Model file for the job. Use its own axes, mm. Round coordinates to 2 decimals unless told otherwise and drop trailing zeros. Loops run counter-clockwise (first coordinate to the right, second up) from the corner with the lowest first, then second, coordinate; pieces in that order, holes last. Notation, with made-up numbers: (59, 82) -> (91, 82) arc R13 ccw to (91, 103) -> close; hole circle Ø7 at (18.5, 48). An arc over 180 degrees is marked (long way). Use a Markdown table: item, result.
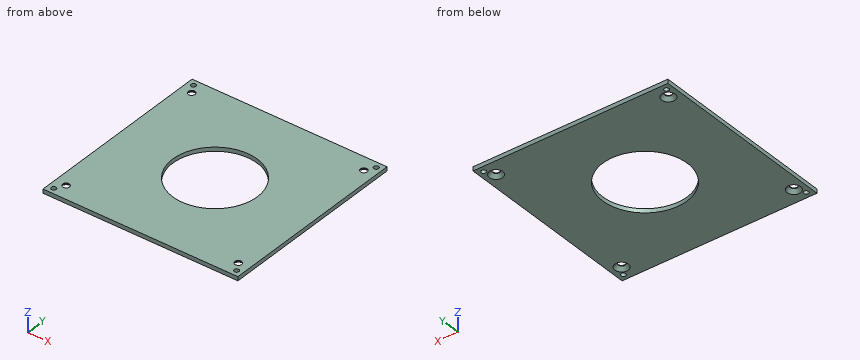
from build123d import *

# Parameters (mm, degrees)
PLATE_SKETCH_W                 = 97
PLATE_SKETCH_H                 = 95
PLATE_DEPTH                    = 2
M2_FOOT_SCREW_HOLES_DEPTH      = 136.786597277
M2_FOOT_SCREW_HOLES_DEPTH_BACK = 136.786597277
M2_FOOT_SCREW_HOLES_SKETCH_R   = 1.2
M3_STACK_ROD_HOLES_DEPTH       = 136.786597277
M3_STACK_ROD_HOLES_DEPTH_BACK  = 136.786597277
M3_STACK_ROD_HOLES_SKETCH_R    = 1.7
M3_COUNTERSINKS_SIZE           = 1.66
CAMERA_APERTURE_DEPTH          = 136.786597277
CAMERA_APERTURE_DEPTH_BACK     = 136.786597277
CAMERA_APERTURE_SKETCH_R       = 21


with BuildPart() as part:
    # Plate sketch → Plate (new body)
    with BuildSketch(Plane.XY):
        with Locations((48.5, 47.5)):
            Rectangle(PLATE_SKETCH_W, PLATE_SKETCH_H)
    extrude(amount=PLATE_DEPTH)

    # M2 foot screw holes sketch → M2 foot screw holes (cut, two sides: drawn at the far end of the back side and taken through both)
    with BuildSketch(Plane.XY.offset(-M2_FOOT_SCREW_HOLES_DEPTH_BACK)):
        with Locations((3, 3)):
            Circle(M2_FOOT_SCREW_HOLES_SKETCH_R)
        with Locations((94, 3)):
            Circle(M2_FOOT_SCREW_HOLES_SKETCH_R)
        with Locations((3, 92)):
            Circle(M2_FOOT_SCREW_HOLES_SKETCH_R)
        with Locations((94, 92)):
            Circle(M2_FOOT_SCREW_HOLES_SKETCH_R)
    extrude(amount=M2_FOOT_SCREW_HOLES_DEPTH + M2_FOOT_SCREW_HOLES_DEPTH_BACK, mode=Mode.SUBTRACT)

    # M3 stack rod holes sketch → M3 stack rod holes (cut, two sides: drawn at the far end of the back side and taken through both)
    with BuildSketch(Plane.XY.offset(-M3_STACK_ROD_HOLES_DEPTH_BACK)):
        with Locations((5.635, 7.495)):
            Circle(M3_STACK_ROD_HOLES_SKETCH_R)
        with Locations((91.365, 7.495)):
            Circle(M3_STACK_ROD_HOLES_SKETCH_R)
        with Locations((5.635, 87.505)):
            Circle(M3_STACK_ROD_HOLES_SKETCH_R)
        with Locations((91.365, 87.505)):
            Circle(M3_STACK_ROD_HOLES_SKETCH_R)
    extrude(amount=M3_STACK_ROD_HOLES_DEPTH + M3_STACK_ROD_HOLES_DEPTH_BACK, mode=Mode.SUBTRACT)

    # M3 countersinks
    m3_countersinks_edges = [part.edges().sort_by_distance(p)[0] for p in [
        (89.665, 7.495, 0),
        (3.935, 87.505, 0),
        (89.665, 87.505, 0),
        (3.935, 7.495, 0),
    ]]
    chamfer(m3_countersinks_edges, length=M3_COUNTERSINKS_SIZE)

    # Camera aperture sketch → Camera aperture (cut, two sides: drawn at the far end of the back side and taken through both)
    with BuildSketch(Plane.XY.offset(-CAMERA_APERTURE_DEPTH_BACK)):
        with Locations((48.5, 47.5)):
            Circle(CAMERA_APERTURE_SKETCH_R)
    extrude(amount=CAMERA_APERTURE_DEPTH + CAMERA_APERTURE_DEPTH_BACK, mode=Mode.SUBTRACT)


solid = part.part
Q1. Band-saw the part on B-B, the plane x = 48.5. Give the cut face in (y, z), plus the area to 3 significant figures.
Results list:
| item | result |
|---|---|
| outline | (0, 0) -> (26.5, 0) -> (26.5, 2) -> (0, 2) -> close; (68.5, 0) -> (95, 0) -> (95, 2) -> (68.5, 2) -> close |
| area | 106 mm² |
Q2. Flat gauge pins, fed straight in: pin 1 (3 mm diameter, centred on x = 91.365, y = 7.495, fed in from -Z); pin 2 (3 mm diameter, centred on x = 3, y = 92, fed in from +Z); pin 3 (5.5 mm diameter, centred on x = 5.635, y = 7.495, fed in from -Z). Where does each tip first touch, or does it go through?
Results list:
| item | result |
|---|---|
| pin 1 | passes through |
| pin 2 | stops at z = 2 |
| pin 3 | stops at z = 0.61 |
Q3. Drill centre lines: L1, parallel to X at y = 3, z = 1.2; L2, parallel to Y at x = 3, z = 1.2; L3, parallel to Y at x = 39.5, z = 1. Where is each one in solid material? Low to high. Write a range as from..to.
Results list:
| item | result |
|---|---|
| L1 | x = 0..1.8, 4.2..92.8, 95.2..97 |
| L2 | y = 0..1.8, 4.2..90.8, 93.2..95 |
| L3 | y = 0..28.53, 66.47..95 |
Q4. Band-saw the part on C-C, the plane y = 47.5. Give the cut face in (x, z).
Results list:
| item | result |
|---|---|
| outline | (0, 0) -> (27.5, 0) -> (27.5, 2) -> (0, 2) -> close; (69.5, 0) -> (97, 0) -> (97, 2) -> (69.5, 2) -> close |
Q5. Band-saw the part on D-D, the plane z = 0.75. Give the number of separate pieces and of enclosed holes in the cut face, plus the area to 3 significant figures.
Results list:
| item | result |
|---|---|
| separate pieces | 1 |
| enclosed holes | 9 |
| area | 7,730 mm² |
Q6. Band-saw the part on A-A, the plane y = 92. Give the cut face in (x, z), plus the area to 3 significant figures.
Results list:
| item | result |
|---|---|
| outline | (0, 0) -> (1.8, 0) -> (1.8, 2) -> (0, 2) -> close; (4.2, 0) -> (92.8, 0) -> (92.8, 2) -> (4.2, 2) -> close; (95.2, 0) -> (97, 0) -> (97, 2) -> (95.2, 2) -> close |
| area | 184 mm² |
